The model under review builds one solid part; all positions refer to its coordinate system, in mm. A direction names the side the tool comes from. Give positions to 0.01 mm unless a question says otherwise; leave off trailing zeros. Write each loop counter-clockwise with the first axis right and the second up, starting at its lowest first coordinate (ties: lowest second). Pieces come first, ordered by that corner, then holes. Notation, with made-up numbers: M 12.25,-22.75 L 41.25,-22.75 A15 ccw 41.25,-1.75 Z; hole C 45,82 d9. An arc over 180 degrees is marked long. Write item = value, one per line. Start each with the question number.
```python
from build123d import *

# Parameters (mm, degrees)
BOSS_EXTRUDE2_DEPTH = 800


with BuildPart() as part:
    # Sketch1 → Boss-Extrude2 (new body)
    with BuildSketch(Plane(origin=(0, 0, 0), x_dir=(1, 0, 0), z_dir=(0, 1, 0))):
        with BuildLine():
            Line((-15, 2.5), (15, 2.5))
            ThreePointArc((15, 2.5), (18.535533906, 3.964466094), (20, 7.5))
            Line((20, 7.5), (20, 27.5))
            Line((20, 27.5), (25, 27.5))
            Line((25, 27.5), (25, 2.5))
            ThreePointArc((25, 2.5), (23.535533906, -1.035533906), (20, -2.5))
            Line((20, -2.5), (-20, -2.5))
            ThreePointArc((-20, -2.5), (-23.535533906, -1.035533906), (-25, 2.5))
            Line((-25, 2.5), (-25, 27.5))
            Line((-25, 27.5), (-20, 27.5))
            Line((-20, 27.5), (-20, 7.5))
            ThreePointArc((-20, 7.5), (-18.535533906, 3.964466094), (-15, 2.5))
        make_face()
    extrude(amount=BOSS_EXTRUDE2_DEPTH)


solid = part.part
```
Item 1: To check wall thickness, follow probe 1 along X at (y, z) = (721.5, -16.25); probe 2 along Z at (x, y) = (-11, 561); probe 3 along Z at (x, y) = (23, 762). State the ranges of each line that lie inside material, in increasing order. Write a range as [from, to].
Item 2: The part is to be moulded in two halves that separate along X. For faces 3 (the flat face through (-20, 394, -18)), 4 (the flat face through (-4, 800, -1)), 5 (the flat face through (-25, 394, -15)), 6 (the flat face through (0, 394, -2.5)), say which applies: released by +X, released by -X, zero draft, split by the parting line, or undercut.
Item 3: We need section A-A, the plane z = -12.75. Write out the cut boundary in (x, y).
Item 4: We need section B-B, the plane y = 321. Write out the cut boundary in (x, z).
Item 5: For faces 1 (the flat face through (25, 394, -15)), 2 (the flat face through (20, 394, -17)), list the 3-axis set-ups (+Z, -Z, +X, -X, +Y, -Y) from which the entire face can be reached by the end or side of a thin tool; tool diameter is ignored.
Item 6: Clearance check with flat-ended pins moving along their axes: P1, Ø1.5, axis at x = -16, y = 697, coming from the -Z side; P2, Ø9, axis at x = 2.5, y = 271.5, coming from the -Z side. State where each tip first meets the part, or that it passes through.
Item 7: We need section C-C, the plane x = 5. Write out the cut boundary in (y, z).
Worked out:
q1.probe_1 = [-25, -20], [20, 25]
q1.probe_2 = [-2.5, 2.5]
q1.probe_3 = [-27.5, 1.5]
q2.face_3 = undercut
q2.face_4 = zero draft
q2.face_5 = released by -X
q2.face_6 = undercut
q3.outline = M -25,0 L -20,0 L -20,800 L -25,800 Z; M 20,0 L 25,0 L 25,800 L 20,800 Z
q4.outline = M -25,-27.5 L -20,-27.5 L -20,-7.5 A5 cw -15,-2.5 L 15,-2.5 A5 cw 20,-7.5 L 20,-27.5 L 25,-27.5 L 25,-2.5 A5 ccw 20,2.5 L -20,2.5 A5 ccw -25,-2.5 Z
q5.face_1 = +Z, -Z, +X, +Y, -Y
q5.face_2 = -Z, +Y, -Y
q6.P1 = -2.82
q6.P2 = -2.5
q7.outline = M 0,-2.5 L 800,-2.5 L 800,2.5 L 0,2.5 Z
